Model file for the job. Use its own axes, mm. A direction names the side the tool comes from. Round coordinates to 2 decimals unless told otherwise and drop trailing zeros. Loops run counter-clockwise (first coordinate to the right, second up) from the corner with the lowest first, then second, coordinate; pieces in that order, holes last. Notation, with made-up numbers: M 19,-31.75 L 71,-31.75 A26 ccw 71,1.25 Z; hole C -29,50.25 d10. An arc over 180 degrees is marked long. Use a Markdown table: item, result. Add a question column.
Q1. Mould opens along X. For faces 1 (the face through (-67.6, -13, -29)), 2 (the face through (-53, 0, -34)), 3 (the face through (-80.3, -13, -34)) say: +X half, -X half, draft (parallel to the pull), parting line (faces both ways), or undercut.
Q2. Cut at C-C (y = -13.25). Give the cut face in (x, z).
Q3. Cut at A-A (x = -66). Give the cut face in (y, z).
Q4. Cut at B-B (z = -7). Give the cut face in (x, y).
Q5. Probe line 1 (X direction, y = -20, z = -29); line 2 (Z direction, x = -61, y = -11.75). List the from-to ranges inside material, lowest first. Write a range as from..to.
Q6. Tool access for faces 4 (the face through (-54.971, -13, -28)), 5 (the face through (-61, -13, 9.361)): list every direction of +Z, -Z, +X, -X, +Y, -Y with a clear straight run to the whole face (end or side of a thin tool).
from build123d import *

# Parameters (mm, degrees)
F0_W     = 12.7
F0_H     = 50.8
F1_DEPTH = 25.4


with BuildPart() as f1:
    # F0 (on Front) → F1 (new body)
    with BuildSketch(Plane.XZ):
        Polygon((-80.300115, 9.361282), (-80.300115, -3.338718), (-67.600115, -3.338718), (-54.970883, -3.338718), (-54.900115, -3.338718), (-42.270883, -3.338718), (-42.270883, 9.361282), (-54.900115, 9.361282), (-67.600115, 9.361282), align=None)
        with Locations((-73.950115, -28.738718)):
            Rectangle(F0_W, F0_H)
        Polygon((-54.970883, -3.338718), (-54.970883, -54.138718), (-42.270883, -54.138718), (-42.270883, -3.338718), (-54.900115, -3.338718), align=None)
        Polygon((-67.600115, -54.138718), (-80.300115, -54.138718), (-80.300115, -79.538718), (-42.270883, -79.538718), (-42.270883, -54.138718), (-54.970883, -54.138718), align=None)
    extrude(amount=F1_DEPTH)


solid = f1.part
Checked values:
| question | item | result |
|---|---|---|
| 1 | face 1 | undercut |
| 1 | face 2 | draft |
| 1 | face 3 | -X half |
| 2 | outline | M -80.3,-79.54 L -42.27,-79.54 L -42.27,9.36 L -80.3,9.36 Z; hole M -67.6,-54.14 L -54.97,-54.14 L -54.97,-3.34 L -67.6,-3.34 Z |
| 3 | outline | M -25.4,-79.54 L 0,-79.54 L 0,-54.14 L -25.4,-54.14 Z; M -25.4,-3.34 L 0,-3.34 L 0,9.36 L -25.4,9.36 Z |
| 4 | outline | M -80.3,-25.4 L -67.6,-25.4 L -67.6,0 L -80.3,0 Z; M -54.97,-25.4 L -42.27,-25.4 L -42.27,0 L -54.97,0 Z |
| 5 | line 1 | x = -80.3..-67.6, -54.97..-42.27 |
| 5 | line 2 | z = -79.54..-54.14, -3.34..9.36 |
| 6 | face 4 | +Y, -Y |
| 6 | face 5 | +Z, +X, -X, +Y, -Y |
